Geometry check sheet. Reference: the model listing, model coordinates, mm. Face numbers are marked on the shaded views. A direction names the side the tool comes from. Give positions to 0.01 mm unless a question says otherwise; leave off trailing zeros. Write each loop counter-clockwise with the first axis right and the second up, starting at its lowest first coordinate (ties: lowest second). Pieces come first, ordered by that corner, then holes. Notation, with made-up numbers: (20, 76.25) -> (72, 76.25) arc R15 cw to (72, 97.25) -> close; hole circle Ø10 at (-20.5, 18.25). An arc over 180 degrees is marked (long way). Use a Markdown table: item, result. Add a question column.
from build123d import *

# Parameters (mm, degrees)
SKETCH1_W           = 50
SKETCH1_H           = 20
BOSS_EXTRUDE1_DEPTH = 470
SKETCH2_W           = 150
SKETCH2_H           = 100
BOSS_EXTRUDE2_DEPTH = 20
SKETCH3_W           = 50
SKETCH3_H           = 20
SKETCH3_H_2         = 50
BOSS_EXTRUDE3_DEPTH = 100


with BuildPart() as part:
    # Sketch1 → Boss-Extrude1 (new body)
    with BuildSketch(Plane.XY):
        Rectangle(SKETCH1_W, SKETCH1_H)
    extrude(amount=BOSS_EXTRUDE1_DEPTH)

    # Sketch2 → Boss-Extrude2 (add)
    with BuildSketch(Plane(origin=(0, 10, 0), x_dir=(1, 0, 0), z_dir=(0, 1, 0))):
        with Locations((-20, -420)):
            Rectangle(SKETCH2_W, SKETCH2_H)
    extrude(amount=-BOSS_EXTRUDE2_DEPTH)

    # Sketch3 → Boss-Extrude3 (add)
    with BuildSketch(Plane(origin=(0, 10, 0), x_dir=(1, 0, 0), z_dir=(0, 1, 0))):
        with Locations((0, -20)):
            Rectangle(SKETCH3_W, SKETCH3_H)
        with Locations((0, -270)):
            Rectangle(SKETCH3_W, SKETCH3_H_2)
    extrude(amount=BOSS_EXTRUDE3_DEPTH)


solid = part.part
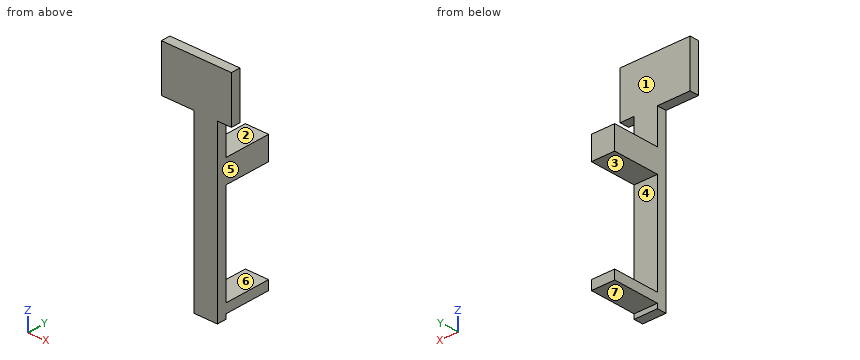
1) Tool access check on the marked faces 5, 6 and 7. Record the directions out of +Z, -Z, +X, -X, +Y, -Y that give a thin tool (end or side, any length) a straight path to the whole face; none if there is none.
2) Sectioned sample at D-D, the plane y = 1. Enter the section's corners in (x, z), and give its area (3 significant figures).
3) Sectioned sample at B-B, the plane x = 0. Enter the section's corners in (y, z).
4) Sectioned sample at A-A, the plane y = 43.5. Enter the section's corners in (x, z).
5) Sectioned sample at C-C, the plane z = 82. Enter the section's corners in (x, y).
6) Gauge pin test, flat ends, axial feed: P1, Ø3, axis at x = -59.5, z = 403, coming from the +Y side; P2, Ø16, axis at x = 41.5, y = -2.5, coming from the -Z side; P3, Ø4, axis at x = -13, y = 67, coming from the -Z side. Record the tip position at first contact, or that the pin passes through.
7) Material ranges on probe 1 along Z at (x, y) = (-6, 12); probe 2 along Y at (x, z) = (-13.5, 200); probe 3 along X at (y, z) = (3, 194), recorded low to high. Write a range as [from, to].
8) Draft check along Z on the marked faces 1, 2, 3 and 4. Enter one of: +Z half, -Z half, draft (parallel to the pull), parting line (faces both ways), or undercut.
Check values:
| question | item | result |
|---|---|---|
| 1 | face 5 | -Z, +X, +Y, -Y |
| 1 | face 6 | +X, -X, +Y |
| 1 | face 7 | -Z, +X, -X, +Y |
| 2 | outline | (-95, 370) -> (-25, 370) -> (-25, 0) -> (25, 0) -> (25, 370) -> (55, 370) -> (55, 470) -> (-95, 470) -> close |
| 2 | area | 33,500 mm² |
| 3 | outline | (-10, 0) -> (10, 0) -> (10, 10) -> (110, 10) -> (110, 30) -> (10, 30) -> (10, 245) -> (110, 245) -> (110, 295) -> (10, 295) -> (10, 470) -> (-10, 470) -> close |
| 4 | outline | (-25, 10) -> (25, 10) -> (25, 30) -> (-25, 30) -> close; (-25, 245) -> (25, 245) -> (25, 295) -> (-25, 295) -> close |
| 5 | outline | (-25, -10) -> (25, -10) -> (25, 10) -> (-25, 10) -> close |
| 6 | P1 | y = 10 |
| 6 | P2 | z = 370 |
| 6 | P3 | z = 10 |
| 7 | probe 1 | [10, 30], [245, 295] |
| 7 | probe 2 | [-10, 10] |
| 7 | probe 3 | [-25, 25] |
| 8 | face 1 | draft |
| 8 | face 2 | +Z half |
| 8 | face 3 | undercut |
| 8 | face 4 | undercut |
